from build123d import *

# Parameters (mm, degrees)
SKETCH4_R          = 1.25
SKETCH4_RX         = 4
SKETCH4_RY         = 2
CUT_EXTRUDE1_DEPTH = 5


with BuildPart() as part:
    # Sketch3 → Revolve1 (revolve)
    with BuildSketch(Plane(origin=(0, 0, 0), x_dir=(1, 0, 0), z_dir=(0, 1, 0))):
        Polygon((10.36932978, 23.4), (8.86932978, 23.4), (8.86932978, 21.4), (-8.61067022, 21.4), (-8.61067022, 18.231946605), (9.211549898, 18.231946605), (12.36932978, 13.417613419), (12.36932978, 8), (15.36932978, 8), (15.36932978, 15), (10.843535586, 21.9), (10.36932978, 21.9), (10.36932978, 22.9), (11.36932978, 22.9), (11.36932978, 23.4), align=None)
    revolve(axis=Axis((-29.774212385, 0, 0), (1, 0, 0)))

    # Sketch4 → Cut-Extrude1 (cut)
    with BuildSketch(Plane(origin=(15.36932978, 0, 0), x_dir=(0, 0, -1), z_dir=(1, 0, 0))):
        with Locations((0, 11.5)):
            Circle(SKETCH4_R)
        with Locations((8.131727984, 8.131727984)):
            Circle(SKETCH4_R)
        with Locations((11.5, 0)):
            Circle(SKETCH4_R)
        with Locations((8.131727984, -8.131727984)):
            Circle(SKETCH4_R)
        with Locations((0, -11.5)):
            Circle(SKETCH4_R)
        with Locations((-8.131727984, -8.131727984)):
            Circle(SKETCH4_R)
        with Locations((-11.5, 0)):
            Circle(SKETCH4_R)
        with Locations((-8.131727984, 8.131727984)):
            Circle(SKETCH4_R)
        with Locations((0, 18.5)):
            Ellipse(SKETCH4_RX, SKETCH4_RY)
        with Locations(Location((17.594545551, 5.716814396), (0, 0, -72))):
            Ellipse(SKETCH4_RX, SKETCH4_RY)
        with Locations(Location((10.874027167, -14.966814396), (0, 0, -144))):
            Ellipse(SKETCH4_RX, SKETCH4_RY)
        with Locations(Location((-10.874027167, -14.966814396), (0, 0, 144))):
            Ellipse(SKETCH4_RX, SKETCH4_RY)
        with Locations(Location((-17.594545551, 5.716814396), (0, 0, 72))):
            Ellipse(SKETCH4_RX, SKETCH4_RY)
    extrude(amount=-CUT_EXTRUDE1_DEPTH, mode=Mode.SUBTRACT)


solid = part.part
Work out the finished part from the listing and answer in its coordinate system (mm). A direction names the side the tool comes from. Round coordinates to 2 decimals unless told otherwise and drop trailing zeros. Loops run counter-clockwise (first coordinate to the right, second up) from the corner with the lowest first, then second, coordinate; pieces in that order, holes last. Notation, with made-up numbers: M 80,18.5 L 110,18.5 A16 ccw 110,32.5 Z; hole C 29.25,-30 d1. An arc over 180 degrees is marked long. One line per question, with ' | ' between items. Start each with the question number.
(1) A tool of negligible diameter and unlimited length cuts with its end or side. For faces 3 (the face through (10.369, -12, 19)), 4 (the face through (13.89, 7.37, -7.14)), 5 (the face through (8.869, -19, -10.3)), from which of +Z, -Z, +X, -X, +Y, -Y can it reach the whole face along a straight path? Write none if from no direction.
(2) Flat-ended cylindrical pins translate along their axes: pin 1 Ø3 at (y, z) = (-11.5, 0) entering from -X; pin 2 Ø1 at (x, z) = (-0.5, 1) entering from +Y; pin 3 Ø1.2 at (y, z) = (18, -0.5) entering from +X; pin 4 Ø12 at (y, z) = (-13, 11) entering from +X. Find the tip coordinate at first contact, or state that the pin passes through.
(3) For a pull along Y with two mould halves and no side action, classify faces 1 (the face through (-8.611, 10, -16)), 2 (the face through (15.086, -9.39, 12.246)) as released by +Y, released by -Y, zero draft, split by the parting line, or undercut.
(4) Find the intervals of material crossed by line 1 (Y direction, x = 11.75, z = 10.5); line 2 (Y direction, x = 10.65, z = 0); line 3 (Y direction, x = 14.65, z = 0), in increasing order.
(5) A cutting plane is placed at A-A on x = -1.5. Write down the section's boundary in (y, z).
(6) A cutting plane is placed at B-B on y = 0. Give the number of separate pieces and of enclosed holes in the cut face, plus the area to 3 significant figures.
Geometry check:
1) face 3: +X | face 4: +X, -X | face 5: -X
2) pin 1: stops at x = 12.37 | pin 2: stops at y = 21.39 | pin 3: stops at x = 10.37 | pin 4: stops at x = 15.37
3) face 1: zero draft | face 2: undercut
4) line 1: y = -17.63 to -17.46, -12.84 to -9.8, 9.8 to 17.63 | line 2: y = -23.4 to -22.9, -21.9 to -16.04, 16.04 to 16.5, 20.5 to 21.9, 22.9 to 23.4 | line 3: y = -16.1 to -12.75, -10.25 to -8, 8 to 10.25, 12.75 to 16.1
5) outline: C 0,0 d42.8; hole C 0,0 d36.46
6) separate pieces: 4 | enclosed holes: 0 | area: 194 mm²
